The model under review builds one solid part; all positions refer to its coordinate system, in mm. A direction names the side the tool comes from. Give positions to 0.01 mm unless a question says otherwise; leave off trailing zeros. Order: outer loops, then holes, each group sorted by start corner. A loop starts at its lowest first (then second) coordinate and runs counter-clockwise, first axis right, second up. Notation, with made-up numbers: (79.25, -17) - (96.25, -17) arc R9 ccw to (96.25, -4) - close; hole circle Ø3 at (52, 2). An arc over 180 degrees is marked (long way). Put each result on its own line as item: value.
```python
from build123d import *

# Parameters (mm, degrees)
BOSS_EXTRUDE1_DEPTH = 12.7
SKETCH2_R           = 2.5796875
CUT_EXTRUDE1_DEPTH  = 5.08
SKETCH3_R           = 1.984375
CUT_EXTRUDE2_DEPTH  = 5.08
FILLET1_R           = 7.62


with BuildPart() as part:
    # Sketch1 → Boss-Extrude1 (new body)
    with BuildSketch(Plane.XY):
        Polygon((-32.22474981, 0), (5.87525019, 27.681270317), (5.87525019, 0), align=None)
    extrude(amount=BOSS_EXTRUDE1_DEPTH)

    # Sketch2 → Cut-Extrude1 (cut)
    with BuildSketch(Plane.XZ):
        with Locations((-13.17474981, 6.35)):
            Circle(SKETCH2_R)
    extrude(amount=-CUT_EXTRUDE1_DEPTH, mode=Mode.SUBTRACT)

    # Sketch3 → Cut-Extrude2 (cut)
    with BuildSketch(Plane(origin=(-11.13337724, 15.323779146, 0), x_dir=(0.8090169943749507, 0.5877852522924687, 0), z_dir=(-0.5877852522924687, 0.8090169943749507, 0))):
        with Locations(Location((-2.471180293, -6.35, 0), (0, 0, 180))):
            Circle(SKETCH3_R)
    extrude(amount=-CUT_EXTRUDE2_DEPTH, mode=Mode.SUBTRACT)

    # Fillet1
    fillet1_edges = [part.edges().sort_by_distance(p)[0] for p in [
        (5.87525019, 27.681270317, 6.35),
    ]]
    fillet(fillet1_edges, radius=FILLET1_R)


solid = part.part
```
(1) Take a section at B-B, the plane y = 15.5. Write out the cut boundary in (x, z).
The answers:
outline: (-10.89, 0) - (5.35, 0) - (5.35, 12.7) - (-10.89, 12.7) - close
(2) The part is to be moulded in two halves that separate along Y. For faces 1 (the flat face through (-10.12, 9.78, 6.38)), 2 (the flat face through (-9, 8, 12.7)), 3 (the cylindrical face through (1.61, 19.57, 6.44)), say which applies: pulls with the +Y half, pulls with the -Y half, needs draft (parallel to the pull), parting line crosses it, or undercut.
The answers:
face 1: undercut
face 2: needs draft
face 3: pulls with the +Y half
(3) Wall thickness on L1, parallel to X at y = 11, z = 5.5; L2, parallel to X at y = 4, z = 7.25; L3, parallel to Y at x = -15, z = 3.25: over which ranges is each line inside the solid? List them lowest first.
The answers:
L1: -17.08 to -13.26, -8.83 to 5.88
L2: -26.72 to -15.59, -10.76 to 5.88
L3: 0 to 12.51
(4) Take a section at C-C, the plane x = -24. Write out the cut boundary in (y, z).
The answers:
outline: (0, 0) - (5.98, 0) - (5.98, 12.7) - (0, 12.7) - close
(5) Take a section at A-A, the plane z = 6.35. Write out the cut boundary in (x, y).
The answers:
outline: (-32.22, 0) - (-15.75, 0) - (-15.75, 5.08) - (-10.6, 5.08) - (-10.6, 0) - (5.88, 0) - (5.88, 12.73) arc R7.62 ccw to (-6.22, 18.89) - (-11.53, 15.04) - (-8.54, 10.93) - (-11.75, 8.6) - (-14.74, 12.7) - close
(6) Clearance check with flat-ended pins moving along their axes: pin 1 Ø10 at (x, y) = (-24.5, 15.5) entering from -Z; pin 2 Ø1 at (y, z) = (12.5, 10.5) entering from -X; pin 3 Ø4 at (x, z) = (-13.17, 6.35) entering from +Y; pin 4 Ø1 at (y, z) = (15.5, 10) entering from -X. State where each tip first meets the part, or that it passes through.
The answers:
pin 1: through
pin 2: x = -15.71
pin 3: y = 15.3
pin 4: x = -11.58
(7) For faces 4 (the flat face through (5.875, 6, 6)), 5 (the cylindrical face through (-13.73, 2.5, 3.83)), list the 3-axis set-ups (+Z, -Z, +X, -X, +Y, -Y) from which the entire face can be reached by the end or side of a thin tool; tool diameter is ignored.
The answers:
face 4: +Z, -Z, +X, +Y, -Y
face 5: -Y
